from build123d import *

# Parameters (mm, degrees)
MIEMBRO_ESTRUCTURAL1_DEPTH    = 374.6
CORTAR_EXTRUIR2_DEPTH         = 196.288143284
TALADRO_DE_MARGEN_PARA_1_41_D = 6.7564
SKETCH2_R                     = 4.1671875
CUT_EXTRUDE2_DEPTH            = 3


with BuildPart() as part:
    # Sketch1 → Miembro estructural1 (new body)
    with BuildSketch(Plane.XY.offset(-193.229032258)):
        with BuildLine():
            Line((0, 0), (0, 20))
            ThreePointArc((0, 20), (2.121320344, 19.121320344), (3, 17))
            Line((3, 17), (3, 6.5))
            ThreePointArc((3, 6.5), (4.025126266, 4.025126266), (6.5, 3))
            Line((6.5, 3), (17, 3))
            ThreePointArc((17, 3), (19.121320344, 2.121320344), (20, 0))
            Line((20, 0), (0, 0))
        make_face()
    extrude(amount=MIEMBRO_ESTRUCTURAL1_DEPTH)

    # Croquis2 → Cortar-Extruir2 (cut, through all)
    with BuildSketch(Plane.YZ):
        with BuildLine():
            Line((12.119137035, 168.589088943), (20, 168.589088943))
            Line((20, 168.589088943), (20, 181.370967742))
            Line((20, 181.370967742), (0, 181.370967742))
            ThreePointArc((0, 181.370967742), (3.51143052, 172.56401157), (12.119137035, 168.589088943))
        make_face()
        with BuildLine():
            Line((22.851984592, -180.447153459), (12.119137035, -180.447153459))
            ThreePointArc((12.119137035, -180.447153459), (3.51143052, -184.422076086), (0, -193.229032258))
            Line((0, -193.229032258), (0, -196.975216041))
            Line((0, -196.975216041), (22.851984592, -196.975216041))
            Line((22.851984592, -196.975216041), (22.851984592, -180.447153459))
        make_face()
    extrude(amount=CORTAR_EXTRUIR2_DEPTH, mode=Mode.SUBTRACT)

    # Taladro de margen para 1/41 (through all)
    with Locations(Plane(origin=(0, 0, 0), x_dir=(-1, 0, 0), z_dir=(0, -1, 0))):
        with Locations((-10, -81.370967742), (-10, 93.229032258)):
            Hole(TALADRO_DE_MARGEN_PARA_1_41_D / 2)

    # Sketch2 → Cut-Extrude2 (cut)
    with BuildSketch(Plane.XZ):
        with Locations(Location((10, -40.529032258, 0), (0, 0, 270))):
            Circle(SKETCH2_R)
        with Locations(Location((10, 39.470967742, 0), (0, 0, 270))):
            Circle(SKETCH2_R)
        with Locations(Location((10, 119.470967742, 0), (0, 0, 270))):
            Circle(SKETCH2_R)
        with Locations(Location((10, -120.529032258, 0), (0, 0, 270))):
            Circle(SKETCH2_R)
    extrude(amount=-CUT_EXTRUDE2_DEPTH, mode=Mode.SUBTRACT)


solid = part.part
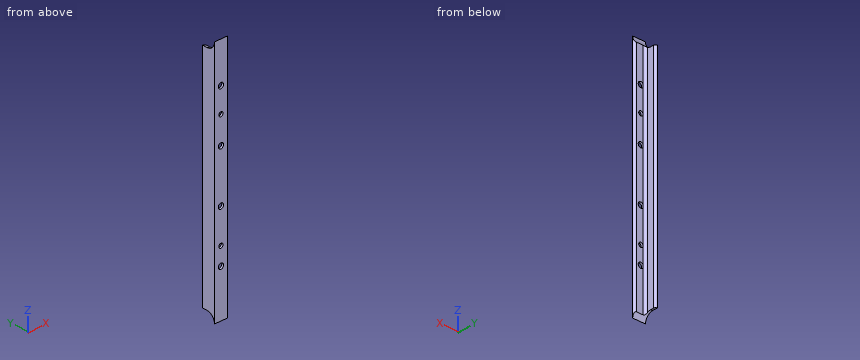
Part model, mm, in its own coordinate system. Round coordinates to 2 decimals unless told otherwise and drop trailing zeros. Loops run counter-clockwise (first coordinate to the right, second up) from the corner with the lowest first, then second, coordinate; pieces in that order, holes last. Notation, with made-up numbers: (16, -36) - (59, -36) arc R33 cw to (59, -5) - close; hole circle Ø2 at (-10, 15). An arc over 180 degrees is marked (long way). Answer as a JSON object with one key per item and string values.
Item 1: Band-saw the part on A-A on x = 10. List the corners of the cut face in (y, z).
Output:
{"outline": "(0, -193.23) arc R12.8 cw to (3, -184.99) - (3, -124.7) - (0, -124.7) - close; (0, -116.36) - (3, -116.36) - (3, -96.61) - (0, -96.61) - close; (0, -89.85) - (3, -89.85) - (3, -44.7) - (0, -44.7) - close; (0, -36.36) - (3, -36.36) - (3, 35.3) - (0, 35.3) - close; (0, 43.64) - (3, 43.64) - (3, 77.99) - (0, 77.99) - close; (0, 84.75) - (3, 84.75) - (3, 115.3) - (0, 115.3) - close; (0, 123.64) - (3, 123.64) - (3, 173.14) arc R12.8 cw to (0, 181.37) - close"}
Item 2: Pin check, flat tips, straight feed: pin 1 (11.5 mm diameter, centred on x = 11, z = 41.5, fed in from +Y); pin 2 (6.5 mm diameter, centred on x = 10, z = 39.47, fed in from -Y); pin 3 (2.5 mm diameter, centred on x = 2, y = 17, fed in from -Z); pin 4 (3 mm diameter, centred on y = 12, z = 3.5, fed in from +X). Stop position of each tip, or through.
Output:
{"pin 1": "y = 3.23", "pin 2": "through", "pin 3": "z = -180.45", "pin 4": "x = 3"}
Item 3: Band-saw the part on B-B on z = 1. List the corners of the cut face in (x, y).
Output:
{"outline": "(0, 0) - (20, 0) arc R3 ccw to (17, 3) - (6.5, 3) arc R3.5 cw to (3, 6.5) - (3, 17) arc R3 ccw to (0, 20) - close"}
Item 4: Wall check: L1, parallel to X at y = 14.5, z = -79.5; L2, parallel to Y at x = 19, z = 140. Give the ranges that are in metal, low to high.
Output:
{"L1": "0 to 3", "L2": "0 to 2.24"}
